Read the model definition and answer for the solid it produces. Units are mm, in the model's axes. A direction names the side the tool comes from. Give positions to 0.01 mm unless a question says otherwise; leave off trailing zeros. Loops run counter-clockwise (first coordinate to the right, second up) from the corner with the lowest first, then second, coordinate; pieces in that order, holes last. Notation, with made-up numbers: (54, 30.25) - (79, 30.25) arc R37 cw to (79, 68.25) - close; hole circle Ø2 at (56, 30). An arc over 180 degrees is marked (long way). Write each question's results on one line, items separated by ' | '. Start each with the question number.
Q1. Given pin 1 (0.9 mm diameter, centred on x = 20.5, z = 168.5, fed in from -Y); pin 2 (2 mm diameter, centred on x = 10.5, y = 2, fed in from +Z); pin 3 (3 mm diameter, centred on x = 56.5, z = 135.5, fed in from -Y), each flat-ended and moving along its own axis, determine where each tip first touches the part or whether it passes through.
Q2. Determine the mould class of faces 4 (the flat face through (10, 1.26, 149)), 5 (the cylindrical face through (67.745, 4.274, 130.509)), 6 (the cylindrical face through (69.574, 4.246, 173.214)) for opening direction Z: +Z half, -Z half, draft (parallel to the pull), parting line (faces both ways), or undercut.
Q3. The part is cut by section A-A, the plane x = 64. Write down the section's boundary in (y, z), plus the area to 3 significant figures.
Q4. The part is cut by section D-D, the plane z = 150. Write down the section's boundary in (x, y).
Q5. Find the intervals of material crossed by line 1 (X direction, y = 2.4, z = 137); line 2 (X direction, y = 4.8, z = 167); line 3 (Y direction, x = 35, z = 143), in increasing order. Write a range as from..to.
Q6. The part is cut by section C-C, the plane y = 4.6. State how many separate pieces and enclosed holes the cut face has, plus the area to 3 significant figures.
Q7. The part is cut by section B-B, the plane z = 130.5. Write down the section's boundary in (x, y), plus the area to 3 significant figures.
Q8. For faces 1 (the cylindrical face through (28.388, 2.767, 165.134)), 2 (the flat face through (28, 2.26, 142)), 3 (the flat face through (9, 2, 163.102)), determine the directions among +Z, -Z, +X, -X, +Y, -Y from which every point of the face is accessible in a straight line to the end or side of a thin tool.
```python
from build123d import *

# Parameters (mm, degrees)
SKETCH1_W           = 66
SKETCH1_H           = 51
SKETCH1_R           = 3
SKETCH1_R_2         = 0.837405072
SKETCH1_R_3         = 0.764054199
SKETCH1_R_4         = 0.803226567
SKETCH1_R_5         = 0.673310758
SKETCH1_R_6         = 0.589146913
BOSS_EXTRUDE1_DEPTH = 2
FILLET1_R           = 3.8
SKETCH2_W           = 5.836445367
SKETCH2_H           = 28.608084639
BOSS_EXTRUDE2_DEPTH = 1
SKETCH3_W           = 4.344585264
SKETCH3_H           = 28.608084639
BOSS_EXTRUDE3_DEPTH = 1
SKETCH4_R           = 1.622882134
SKETCH4_W           = 1.146541205
SKETCH4_H           = 3.7676464
SKETCH4_W_2         = 10.495224563
SKETCH4_H_2         = 14.476262407
SKETCH4_W_3         = 2.954262821
SKETCH4_H_3         = 4.462113597
SKETCH4_W_4         = 4.942556884
SKETCH4_H_4         = 3.116266577
SKETCH4_W_5         = 1.293345918
SKETCH4_H_5         = 3.748296022
BOSS_EXTRUDE4_DEPTH = 1


with BuildPart() as part:
    # Sketch1 → Boss-Extrude1 (new body)
    with BuildSketch(Plane.XZ.offset(-5.259536096)):
        with Locations((37.716985738, 148.797755553)):
            Rectangle(SKETCH1_W, SKETCH1_H)
        with Locations(Location((65.716985738, 128.297755553, 0), (0, 0, 270))):  # turned: the seam where the file's is
            Circle(SKETCH1_R, mode=Mode.SUBTRACT)
        with Locations(Location((9.716985738, 128.297755553, 0), (0, 0, 90))):  # turned: the seam where the file's is
            Circle(SKETCH1_R, mode=Mode.SUBTRACT)
        with Locations(Location((65.716985738, 169.297755553, 0), (0, 0, 90))):  # turned: the seam where the file's is
            Circle(SKETCH1_R, mode=Mode.SUBTRACT)
        with Locations(Location((9.716985738, 169.297755553, 0), (0, 0, 270))):  # turned: the seam where the file's is
            Circle(SKETCH1_R, mode=Mode.SUBTRACT)
        with Locations(Location((60.981346955, 125.297755553, 0), (0, 0, 270))):  # turned: the seam where the file's is
            Circle(SKETCH1_R_2, mode=Mode.SUBTRACT)
        with Locations(Location((58.981346955, 125.297755553, 0), (0, 0, 270))):  # turned: the seam where the file's is
            Circle(SKETCH1_R_2, mode=Mode.SUBTRACT)
        with Locations(Location((56.981346955, 125.297755553, 0), (0, 0, 270))):  # turned: the seam where the file's is
            Circle(SKETCH1_R_2, mode=Mode.SUBTRACT)
        with Locations(Location((54.981346955, 125.297755553, 0), (0, 0, 270))):  # turned: the seam where the file's is
            Circle(SKETCH1_R_2, mode=Mode.SUBTRACT)
        with Locations(Location((56.981346955, 172.297755553, 0), (0, 0, 270))):  # turned: the seam where the file's is
            Circle(SKETCH1_R_3, mode=Mode.SUBTRACT)
        with Locations(Location((54.981346955, 172.297755553, 0), (0, 0, 270))):  # turned: the seam where the file's is
            Circle(SKETCH1_R_4, mode=Mode.SUBTRACT)
        with Locations(Location((7.14174105, 132.13483961, 0), (0, 0, 270))):  # turned: the seam where the file's is
            Circle(SKETCH1_R_5, mode=Mode.SUBTRACT)
        with Locations(Location((7.14174105, 134.559866184, 0), (0, 0, 270))):  # turned: the seam where the file's is
            Circle(SKETCH1_R_6, mode=Mode.SUBTRACT)
    extrude(amount=BOSS_EXTRUDE1_DEPTH)

    # Fillet1
    fillet1_edges = [part.edges().sort_by_distance(p)[0] for p in [
        (70.716985738, 4.259536096, 123.297755553),
        (4.716985738, 4.259536096, 123.297755553),
        (4.716985738, 4.259536096, 174.297755553),
        (70.716985738, 4.259536096, 174.297755553),
    ]]
    fillet(fillet1_edges, radius=FILLET1_R)

    # Sketch2 → Boss-Extrude2 (add)
    with BuildSketch(Plane.XZ.offset(-3.259536096)):
        with Locations((9.268800109, 148.797755553)):
            Rectangle(SKETCH2_W, SKETCH2_H)
    extrude(amount=BOSS_EXTRUDE2_DEPTH)

    # Sketch3 → Boss-Extrude3 (add)
    with BuildSketch(Plane.XZ.offset(-2.259536096)):
        with Locations((10.01473016, 148.797755553)):
            Rectangle(SKETCH3_W, SKETCH3_H)
    extrude(amount=BOSS_EXTRUDE3_DEPTH)

    # Sketch4 → Boss-Extrude4 (add)
    with BuildSketch(Plane.XZ.offset(-3.259536096)):
        with Locations(Location((29.756180169, 164.261204908, 0), (0, 0, 90))):  # turned: the seam where the file's is
            Circle(SKETCH4_R)
        with Locations((52.18819816, 159.346174618)):
            Rectangle(SKETCH4_W, SKETCH4_H)
        with Locations((28.060742514, 141.548791384)):
            Rectangle(SKETCH4_W_2, SKETCH4_H_2)
        with Locations((20.678530081, 167.750382062)):
            Rectangle(SKETCH4_W_3, SKETCH4_H_3)
        with Locations((52.621525564, 169.30851535)):
            Rectangle(SKETCH4_W_4, SKETCH4_H_4)
        with Locations((54.18819816, 159.346174618)):
            Rectangle(SKETCH4_W, SKETCH4_H)
        with Locations((50.18819816, 159.346174618)):
            Rectangle(SKETCH4_W, SKETCH4_H)
        with Locations((48.18819816, 159.346174618)):
            Rectangle(SKETCH4_W, SKETCH4_H)
        with Locations((46.18819816, 159.346174618)):
            Rectangle(SKETCH4_W, SKETCH4_H)
        with Locations((44.18819816, 159.346174618)):
            Rectangle(SKETCH4_W, SKETCH4_H)
        with Locations((42.18819816, 159.346174618)):
            Rectangle(SKETCH4_W, SKETCH4_H)
        with Locations((40.18819816, 159.346174618)):
            Rectangle(SKETCH4_W, SKETCH4_H)
        with Locations((38.18819816, 159.346174618)):
            Rectangle(SKETCH4_W, SKETCH4_H)
        with Locations((36.18819816, 159.346174618)):
            Rectangle(SKETCH4_W, SKETCH4_H)
        with Locations((22.523111138, 126.647676881)):
            Rectangle(SKETCH4_W_5, SKETCH4_H_5)
        with Locations((17.523111138, 126.647676881)):
            Rectangle(SKETCH4_W_5, SKETCH4_H_5)
        with Locations((27.523111138, 126.647676881)):
            Rectangle(SKETCH4_W_5, SKETCH4_H_5)
        with Locations((32.523111138, 126.647676881)):
            Rectangle(SKETCH4_W_5, SKETCH4_H_5)
        with Locations((37.523111138, 126.647676881)):
            Rectangle(SKETCH4_W_5, SKETCH4_H_5)
    extrude(amount=BOSS_EXTRUDE4_DEPTH)


solid = part.part
```
Check sheet entries:
1) pin 1: stops at y = 2.26 | pin 2: stops at z = 163.1 | pin 3: stops at y = 3.26
2) face 4: draft | face 5: undercut | face 6: +Z half
3) outline: (3.26, 123.3) - (5.26, 123.3) - (5.26, 125.84) - (3.26, 125.84) - close; (3.26, 130.76) - (5.26, 130.76) - (5.26, 166.84) - (3.26, 166.84) - close; (3.26, 171.76) - (5.26, 171.76) - (5.26, 174.3) - (3.26, 174.3) - close | area: 82.3 mm^2
4) outline: (4.72, 3.26) - (6.35, 3.26) - (6.35, 2.26) - (7.84, 2.26) - (7.84, 1.26) - (12.19, 1.26) - (12.19, 3.26) - (70.72, 3.26) - (70.72, 5.26) - (4.72, 5.26) - close
5) line 1: x = 6.35..12.19, 22.81..33.31 | line 2: x = 4.72..7.79, 11.65..63.79, 67.65..70.72 | line 3: y = 3.26..5.26
6) separate pieces: 1 | enclosed holes: 12 | area: 3,230 mm^2
7) outline: (4.72, 3.26) - (7.68, 3.26) - (7.68, 5.26) - (4.72, 5.26) - close; (11.75, 3.26) - (63.68, 3.26) - (63.68, 5.26) - (11.75, 5.26) - close; (67.75, 3.26) - (70.72, 3.26) - (70.72, 5.26) - (67.75, 5.26) - close | area: 116 mm^2
8) face 1: -Y | face 2: +Z, -Z, +X, -Y | face 3: +Z, -X, -Y
